Geometry check sheet. Reference: the model listing, model coordinates, mm. Give positions to 0.01 mm unless a question says otherwise; leave off trailing zeros. Loops run counter-clockwise (first coordinate to the right, second up) from the corner with the lowest first, then second, coordinate; pieces in that order, holes last.
1. Cross-section at B-B, the plane z = 18.5. Record the cut outline in (x, y).
2. Go/stop test with flat-tipped pins: pin 1 Ø1.5 at (y, z) = (1, 14) entering from -X; pin 2 Ø1 at (x, z) = (-1, 12) entering from -Y. Record where each tip stops, or that it passes through.
3. Cross-section at A-A, the plane x = 0. Record the cut outline in (y, z), plus the area to 3 significant figures.
4. Material ranges on L1, parallel to Z at x = 0, y = -1.2; L2, parallel to Z at x = 2, y = 1.75; L3, parallel to X at y = 1.5, z = 18, recorded low to high.
5. Cross-section at C-C, the plane z = 25. Record the cut outline in (x, y), plus the area to 3 significant figures.
from build123d import *

# Parameters (mm, degrees)
F0_R          = 4.699
F1_DEPTH      = 31.7754
F2_R          = 3.175
F3_DEPTH      = 14.986
F3_DEPTH_BACK = 25.4
F4_R          = 0.79375


with BuildPart() as f1:
    # F0 (on Top) → F1 (new body)
    with BuildSketch(Plane.XY):
        Circle(F0_R)
    extrude(amount=F1_DEPTH)

    # F2 (on Front) → F3 (cut, two sides)
    with BuildSketch(Plane.XZ) as f3_sk:
        with Locations((0, 15.875)):
            Circle(F2_R)
    extrude(amount=-F3_DEPTH, mode=Mode.SUBTRACT)
    extrude(f3_sk.sketch, amount=F3_DEPTH_BACK, mode=Mode.SUBTRACT)

    # F4
    f4_edges = [f1.edges().sort_by_distance(p)[0] for p in [
        (-4.699, 0, 31.7754),
        (-4.699, 0, 0),
    ]]
    fillet(f4_edges, radius=F4_R)


solid = f1.part
Result:
1. outline: (-1.79, -4.35) - (-1.79, 4.35) arc R4.7 ccw to start; (1.79, -4.35) arc R4.7 ccw to (1.79, 4.35) - close
2. pin 1: stops at x = -4.69
2. pin 2: stops at y = -4.67
3. outline: (-4.7, 0.79) arc R0.79 ccw to (-3.91, 0) - (3.91, 0) arc R0.79 ccw to (4.7, 0.79) - (4.7, 12.7) - (-4.7, 12.7) - close; (-4.7, 19.05) - (4.7, 19.05) - (4.7, 30.98) arc R0.79 ccw to (3.91, 31.78) - (-3.91, 31.78) arc R0.79 ccw to (-4.7, 30.98) - close
3. area: 238 mm2
4. L1: z = 0 to 12.7, 19.05 to 31.78
4. L2: z = 0 to 13.41, 18.34 to 31.78
4. L3: x = -4.45 to -2.36, 2.36 to 4.45
5. outline: circle Ø9.4 at (0, 0)
5. area: 69.4 mm2
